Job drawing, mm, ordinate dimensions from the low corner. One solid piece. A direction names the side the tool comes from. Coordinates: 2 decimals unless noted, no trailing zeros. Write each loop counter-clockwise with the first axis right and the second up, starting at its lowest first coordinate (ties: lowest second). Pieces come first, ordered by that corner, then holes. Notation, with made-up numbers: (58, 26.5) - (107, 26.5) arc R16 cw to (107, 37.5) - close; hole circle Ø8 at (-33, -38). An arc over 180 degrees is marked (long way). Put each result on its own line as item: value. Start each with the question number.
1. Pull direction Z, two halves, no side cores. Call the marked faces 1, 2 and 3: released by +Z, released by -Z, zero draft, split by the parting line, or undercut.
2. Drill centre lines: L1, parallel to X at y = 4.75, z = 33; L2, parallel to X at y = 1, z = 4; L3, parallel to Z at x = 19.5, y = 2.5. Where is each one in solid material? Low to high. Write a range as from..to.
3. Saw through at B-B, the plane y = 1. Write the cut outline in (x, z).
4. Drop flat-ended pins along their axis: P1, Ø1.5, axis at y = 3.5, z = 28.5, coming from the -X side; P2, Ø3, axis at x = 8.5, y = 4, coming from the +Z side; P3, Ø1.5, axis at y = 3.5, z = 4, coming from the +X side. Give the stop position or say it passes through.
5. Which spindle directions (+Z, -Z, +X, -X, +Y, -Y) get a long thin tool onto all of the face, cutting with end or side? Do the marked faces 4, 5 and 6. Say none if no direction does.
6. Saw through at A-A, the plane z = 2.5. Write the cut outline in (x, y), plus the area to 4 significant figures.
7. Saw through at C-C, the plane x = 24. Write the cut outline in (y, z), plus the area to 3 significant figures.
8. Saw through at D-D, the plane z = 17. Write the cut outline in (x, y).
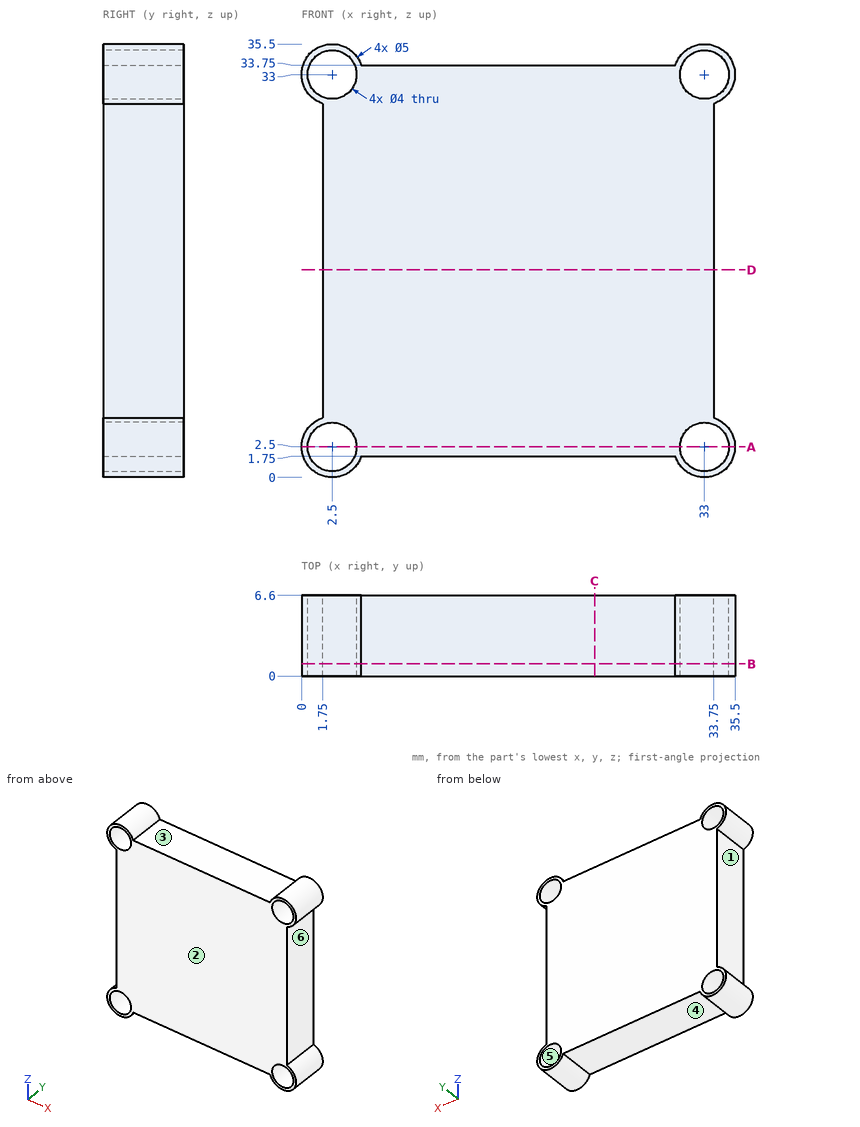
Final values:
1. face 1: undercut
1. face 2: zero draft
1. face 3: released by +Z
2. L1: x = 0..0.5, 4.5..31, 35..35.5
2. L2: x = 0.5..1.18, 3.82..31.68, 34.32..35
2. L3: z = 1.75..33.75
3. outline: (1.75, 4.88) arc R2.5 ccw (long way) to (4.88, 1.75) - (30.62, 1.75) arc R2.5 ccw (long way) to (33.75, 4.88) - (33.75, 30.62) arc R2.5 ccw (long way) to (30.62, 33.75) - (4.88, 33.75) arc R2.5 ccw (long way) to (1.75, 30.62) - close; hole circle Ø4 at (2.5, 2.5); hole circle Ø4 at (2.5, 33); hole circle Ø4 at (33, 2.5); hole circle Ø4 at (33, 33)
4. P1: stops at x = 1.75
4. P2: stops at z = 33.75
4. P3: stops at x = 35.38
5. face 4: -Z, +Y, -Y
5. face 5: +Y, -Y
5. face 6: +X, +Y, -Y
6. outline: (0, 0) - (0.5, 0) - (0.5, 6.6) - (0, 6.6) - close; (4.5, 0) - (31, 0) - (31, 6.6) - (4.5, 6.6) - close; (35, 0) - (35.5, 0) - (35.5, 6.6) - (35, 6.6) - close
6. area: 181.5 mm²
7. outline: (0, 1.75) - (6.6, 1.75) - (6.6, 33.75) - (0, 33.75) - close
7. area: 211 mm²
8. outline: (1.75, 0) - (33.75, 0) - (33.75, 6.6) - (1.75, 6.6) - close
